Read the model definition and answer for the solid it produces. Units are mm, in the model's axes. Coordinates: 2 decimals unless noted, no trailing zeros. Order: outer loops, then holes, each group sorted by start corner. A loop starts at its lowest first (then second) coordinate and runs counter-clockwise, first axis right, second up.
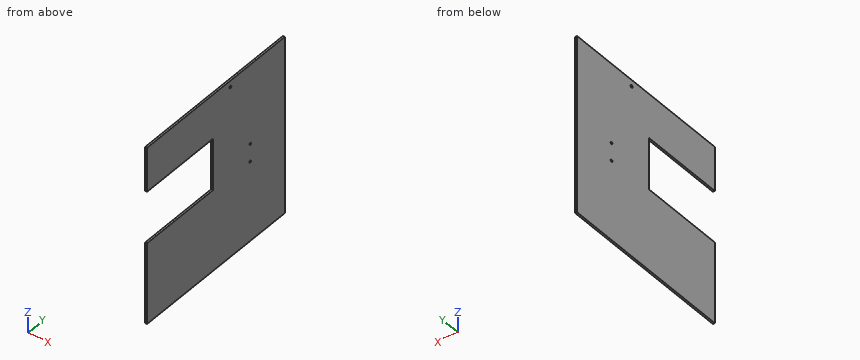
```python
from build123d import *

# Parameters (mm, degrees)
BOSS_EXTRUDE1_DEPTH       = 3.175
SKETCH2_R                 = 2.286
CUT_EXTRUDE1_DEPTH        = 216.549531721
F_6_0_15_DIAMETER_HOLE1_D = 3.81


with BuildPart() as part:
    # Sketch1 → Boss-Extrude1 (new body)
    with BuildSketch(Plane(origin=(0, 0, 0), x_dir=(0, 0, -1), z_dir=(1, 0, 0))):
        Polygon((152.4, 152.4), (-152.4, 152.4), (-152.4, -152.4), (-76.2, -152.4), (-76.2, -6.35), (12.7, -6.35), (12.7, -152.4), (152.4, -152.4), align=None)
    extrude(amount=BOSS_EXTRUDE1_DEPTH)

    # Sketch2 → Cut-Extrude1 (cut, through all)
    with BuildSketch(Plane(origin=(3.175, 0, 0), x_dir=(0, 0, -1), z_dir=(1, 0, 0))):
        with Locations((-141.2875, 31.75)):
            Circle(SKETCH2_R)
    extrude(amount=-CUT_EXTRUDE1_DEPTH, mode=Mode.SUBTRACT)

    # #6 (0.15) Diameter Hole1 (through all)
    with Locations(Plane(origin=(3.175, 0, 0), x_dir=(0, 0, -1), z_dir=(1, 0, 0))):
        with Locations((-15.24, 76.2), (15.24, 76.2)):
            Hole(F_6_0_15_DIAMETER_HOLE1_D / 2)


solid = part.part
```
1) A flat-ended cylindrical pin translates along its axis: pin 1 Ø1.6 at (x, z) = (1, 44) entering from -Y. Find the tip coordinate at first contact, or state that the pin passes through.
A:
pin 1: stops at y = -6.35
2) Straight lines are drawn through the part: line 1 (Z direction, x = 1.4, y = 76.2) (3 decimals); line 2 (Z direction, x = 2.05, y = -27.5); line 3 (Y direction, x = 0.9, z = -15.24) (3 decimals). For each, find the intervals that lie inside material, in ascending order.
A:
line 1: z = -152.4 to -17.145, -13.335 to 13.335, 17.145 to 152.4
line 2: z = -152.4 to -12.7, 76.2 to 152.4
line 3: y = -152.4 to 74.295, 78.105 to 152.4
3) A cutting plane is placed at A-A, the plane y = -133. Determine the outline of the cut face in (x, z) (3 decimals), and give its area (3 significant figures).
A:
outline: (0, -152.4) - (3.175, -152.4) - (3.175, -12.7) - (0, -12.7) - close; (0, 76.2) - (3.175, 76.2) - (3.175, 152.4) - (0, 152.4) - close
area: 685 mm2
4) A cutting plane is placed at B-B, the plane x = 1.9. State how many separate pieces and enclosed holes the cut face has, and give its area (3 significant figures).
A:
separate pieces: 1
enclosed holes: 3
area: 79,900 mm2
